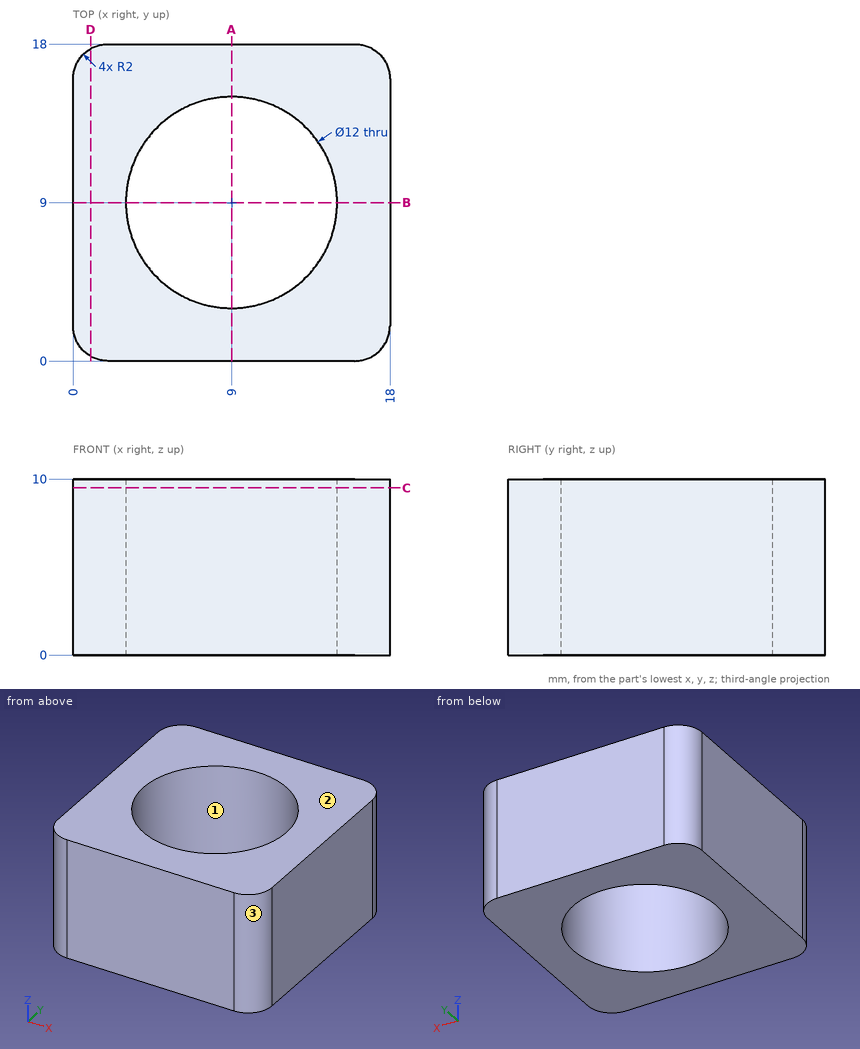
Input: dimensioned drawing with shaded views. Units: mm. Origin: part minimum x, y, z. Give positions to 0.01 mm unless a question says otherwise; leave off trailing zeros. Write each loop counter-clockwise with the first axis right and the second up, starting at its lowest first coordinate (ties: lowest second). Pieces come first, ordered by that corner, then holes.
Q1. Section A-A, the plane x = 9. Output: boundary loops of the cut face in (y, z), plus the area to 3 significant figures.
Q2. Section C-C, the plane z = 9.5. Output: boundary loops of the cut face in (x, y).
Q3. Pull-direction query (X, two-part tool) for the marked faces 1, 2 and 3; classes: pulls with the +X half, pulls with the -X half, needs draft (parallel to the pull), parting line crosses it, or undercut.
Q4. Section D-D, the plane x = 1. Output: boundary loops of the cut face in (y, z), plus the area to 3 significant figures.
Q5. Material intervals for probe 1 along Y at (x, z) = (9, 5.5); probe 2 along Y at (x, z) = (14, 0.75); probe 3 along X at (y, z) = (3.75, 8.75), sorted ascending.
Filled in:
1. outline: (0, 0) - (3, 0) - (3, 10) - (0, 10) - close; (15, 0) - (18, 0) - (18, 10) - (15, 10) - close
1. area: 60.0 mm2
2. outline: (0, 2) arc R2 ccw to (2, 0) - (16, 0) arc R2 ccw to (18, 2) - (18, 16) arc R2 ccw to (16, 18) - (2, 18) arc R2 ccw to (0, 16) - close; hole circle Ø12 at (9, 9)
3. face 1: undercut
3. face 2: needs draft
3. face 3: pulls with the +X half
4. outline: (0.27, 0) - (17.73, 0) - (17.73, 10) - (0.27, 10) - close
4. area: 175 mm2
5. probe 1: y = 0 to 3, 15 to 18
5. probe 2: y = 0 to 5.68, 12.32 to 18
5. probe 3: x = 0 to 6.1, 11.9 to 18
